Source: CAD feature listing. Evaluate the final solid. Frame: model axes, mm. A direction names the side the tool comes from. Round coordinates to 2 decimals unless told otherwise and drop trailing zeros. Loops run counter-clockwise (first coordinate to the right, second up) from the corner with the lowest first, then second, coordinate; pieces in that order, holes last. Notation, with made-up numbers: M 72,-28.5 L 86,-28.5 A11 cw 86,-13.5 Z; hole C -26.5,60 d10. An arc over 180 degrees is marked long. One line per item, written item: value.
from build123d import *

# Parameters (mm, degrees)
SKETCH1_W                                        = 95.25
SKETCH1_H                                        = 63.5
BOSS_EXTRUDE1_DEPTH                              = 12.7
CBORE_FOR_1_4_SOCKET_HEAD_CAP_SCREW1_D           = 7.14248
CBORE_FOR_1_4_SOCKET_HEAD_CAP_SCREW1_CBORE_D     = 11.1125
CBORE_FOR_1_4_SOCKET_HEAD_CAP_SCREW1_CBORE_DEPTH = 6.35
CBORE_FOR_5_8_SOCKET_HEAD_CAP_SCREW1_D           = 16.256
CBORE_FOR_5_8_SOCKET_HEAD_CAP_SCREW1_CBORE_D     = 34.925
CBORE_FOR_5_8_SOCKET_HEAD_CAP_SCREW1_CBORE_DEPTH = 7.9248


with BuildPart() as part:
    # Sketch1 → Boss-Extrude1 (new body)
    with BuildSketch(Plane.XY):
        with Locations((47.625, 31.75)):
            Rectangle(SKETCH1_W, SKETCH1_H)
    extrude(amount=BOSS_EXTRUDE1_DEPTH)

    # CBORE for 1/4 Socket Head Cap Screw1 (through all)
    with Locations(Plane(origin=(0, 0, 0), x_dir=(-1, 0, 0), z_dir=(0, 0, -1))):
        with Locations((-12.7, 53.975), (-12.7, 9.525)):
            CounterBoreHole(CBORE_FOR_1_4_SOCKET_HEAD_CAP_SCREW1_D / 2, CBORE_FOR_1_4_SOCKET_HEAD_CAP_SCREW1_CBORE_D / 2, CBORE_FOR_1_4_SOCKET_HEAD_CAP_SCREW1_CBORE_DEPTH)

    # CBORE for 5/8 Socket Head Cap Screw1 (through all)
    with Locations(Plane.XY.offset(12.7)):
        with Locations((57.15, 31.75)):
            CounterBoreHole(CBORE_FOR_5_8_SOCKET_HEAD_CAP_SCREW1_D / 2, CBORE_FOR_5_8_SOCKET_HEAD_CAP_SCREW1_CBORE_D / 2, CBORE_FOR_5_8_SOCKET_HEAD_CAP_SCREW1_CBORE_DEPTH)


solid = part.part
1. Pin query (flat end, axial travel): pin 1 (10.5 mm diameter, centred on x = 56.5, y = 35, fed in from +Z). Return the tip coordinate at first contact, or that it passes through.
Report:
pin 1: stops at z = 4.78
2. Reachability of faces 1 (the face through (73.28, 25.06, 8.79)), 2 (the face through (0, 31, 6)), 3 (the face through (9, 10, 6.35)) from +Z, -Z, +X, -X, +Y, -Y: full face, straight path, thin tool, end or side. Return the list, or none.
Report:
face 1: +Z
face 2: +Z, -Z, -X, +Y, -Y
face 3: -Z
3. Section query B-B (y = 31.75). Return the cut outline in (x, z), and give its area (3 significant figures).
Report:
outline: M 0,0 L 49.02,0 L 49.02,4.78 L 39.69,4.78 L 39.69,12.7 L 0,12.7 Z; M 65.28,0 L 95.25,0 L 95.25,12.7 L 74.61,12.7 L 74.61,4.78 L 65.28,4.78 Z
area: 855 mm2
4. Pull-direction query (Y, two-part tool) for faces 4 (the face through (95.25, 31, 6)), 5 (the face through (47, 63.5, 6)), 6 (the face through (13.9, 48.55, 3.13)); classes: released by +Y, released by -Y, zero draft, split by the parting line, or undercut.
Report:
face 4: zero draft
face 5: released by +Y
face 6: undercut
5. Ray query, line 1 (Y direction, x = 12.7, z = 2.5); line 2 (Y direction, x = 57.15, z = 9.5); line 3 (X direction, y = 10.5, z = 1). Return the intervals inside material, ascending. Write a range as [from, to].
Report:
line 1: y = [0, 3.97], [15.08, 48.42], [59.53, 63.5]
line 2: y = [0, 14.29], [49.21, 63.5]
line 3: x = [0, 7.23], [18.17, 95.25]
6. Section query C-C (x = 57.15). Return the cut outline in (y, z), and give its area (3 significant figures).
Report:
outline: M 0,0 L 23.62,0 L 23.62,4.78 L 14.29,4.78 L 14.29,12.7 L 0,12.7 Z; M 39.88,0 L 63.5,0 L 63.5,12.7 L 49.21,12.7 L 49.21,4.78 L 39.88,4.78 Z
area: 452 mm2
7. Section query D-D (z = 9). Count the separate pieces of the cut face and the enclosed holes in it, and give its area (3 significant figures).
Report:
separate pieces: 1
enclosed holes: 3
area: 5,010 mm2
8. Section query A-A (x = 12.7). Return the cut outline in (y, z).
Report:
outline: M 0,0 L 3.97,0 L 3.97,6.35 L 5.95,6.35 L 5.95,12.7 L 0,12.7 Z; M 13.1,6.35 L 15.08,6.35 L 15.08,0 L 48.42,0 L 48.42,6.35 L 50.4,6.35 L 50.4,12.7 L 13.1,12.7 Z; M 57.55,6.35 L 59.53,6.35 L 59.53,0 L 63.5,0 L 63.5,12.7 L 57.55,12.7 Z
